Can you work these out from the drawing? Everything is in mm from the part's minimum corner. Give positions to 0.01 mm unless a question says otherwise; leave off trailing zeros. Write each loop counter-clockwise with the first axis right and the second up, starting at its lowest first coordinate (ties: lowest second). Pieces come first, ordered by that corner, then holes. Notation, with made-up numbers: (87, -4) -> (136, -4) arc R18 cw to (136, 20) -> close; hole circle Ø10 at (85.5, 80.5). An arc over 180 degrees is marked (long way). Write item = value, one per line. Start each with the question number.
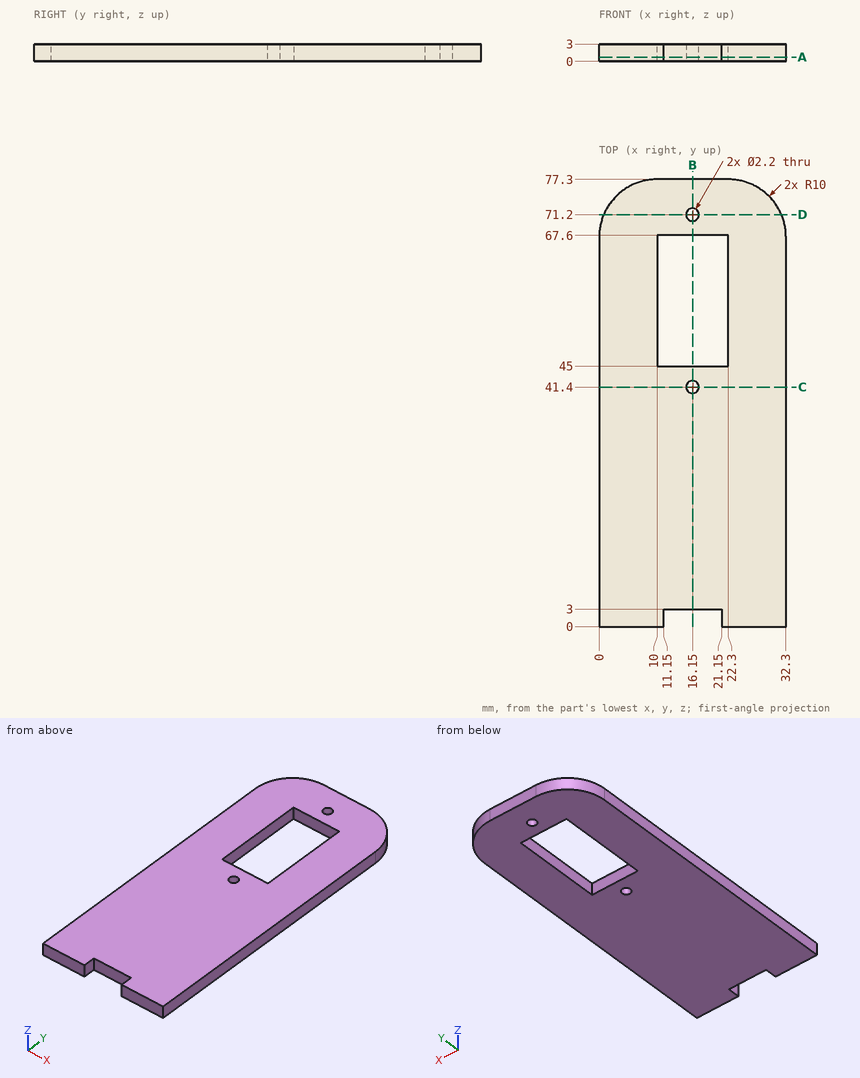
(1) I'm going to push flat-ended pins straight in: pin 1 (5 mm diameter, centred on x = 6.5, y = 8.5, fed in from -Z); pin 2 (1.5 mm diameter, centred on x = 16.5, z = 2, fed in from -Y); pin 3 (1 mm diameter, centred on x = 4.5, z = 2.5, fed in from +Y). Where does each tip first touch, or does it pass through?
(2) Imagine slicing it at B-B (x = 16.15). Please give me the cut outline in (y, z).
(3) Imagine slicing it at C-C (y = 41.4). Please give me the cut outline in (x, z), then the cut area to 3 significant figures.
(4) If I drill on line 1 along Y through (x, z) = (16.15, 2.2); line 2 along Y through (x, z) = (14.5, 1.2); line 3 along X through (y, z) = (53, 1.2), over which ranges is the centre line in solid material (lowest first)? Write a range as from..to.
(5) Imagine slicing it at D-D (y = 71.2). Please give me the cut outline in (x, z).
(6) Imagine slicing it at A-A (z = 0.75). Please give me the cut outline in (x, y).
Answers below:
q1.pin_1 = 0
q1.pin_2 = 3
q1.pin_3 = 75.96
q2.outline = (3, 0) -> (40.3, 0) -> (40.3, 3) -> (3, 3) -> close; (42.5, 0) -> (45, 0) -> (45, 3) -> (42.5, 3) -> close; (67.6, 0) -> (70.1, 0) -> (70.1, 3) -> (67.6, 3) -> close; (72.3, 0) -> (77.3, 0) -> (77.3, 3) -> (72.3, 3) -> close
q3.outline = (0, 0) -> (15.05, 0) -> (15.05, 3) -> (0, 3) -> close; (17.25, 0) -> (32.3, 0) -> (32.3, 3) -> (17.25, 3) -> close
q3.area = 90.3 mm^2
q4.line_1 = 3..40.3, 42.5..45, 67.6..70.1, 72.3..77.3
q4.line_2 = 3..45, 67.6..77.3
q4.line_3 = 0..10, 22.3..32.3
q5.outline = (0.79, 0) -> (15.05, 0) -> (15.05, 3) -> (0.79, 3) -> close; (17.25, 0) -> (31.51, 0) -> (31.51, 3) -> (17.25, 3) -> close
q6.outline = (0, 0) -> (11.15, 0) -> (11.15, 3) -> (21.15, 3) -> (21.15, 0) -> (32.3, 0) -> (32.3, 67.3) arc R10 ccw to (22.3, 77.3) -> (10, 77.3) arc R10 ccw to (0, 67.3) -> close; hole (10, 45) -> (22.3, 45) -> (22.3, 67.6) -> (10, 67.6) -> close; hole circle Ø2.2 at (16.15, 41.4); hole circle Ø2.2 at (16.15, 71.2)
